from build123d import *

# Parameters (mm, degrees)
REVOLUTION_ANGLE = 180


with BuildPart() as part:
    # Sketch → Revolution (revolve)
    with BuildSketch(Plane.XY):
        Polygon((26.5, 9.5), (26.5, 17.46), (19.5, 17.46), (19.5, 18.46), (19, 18.46), (19, 28), (16.5, 28), (16.5, 9), (-19.5, 9), (-19.5, 34), (-22, 34), (-22, 26), (-40, 26), (-40, 9.5), (-50, 9.5), (-50, 2.5), (50, 2.5), (50, 9.5), align=None)
    revolve(axis=Axis((0, 0, 0), (1, 0, 0)), revolution_arc=REVOLUTION_ANGLE)


solid = part.part
For this review, take the finished solid that the model builds, in its own axes (mm). A direction names the side the tool comes from. Coordinates: 2 decimals unless noted, no trailing zeros. Order: outer loops, then holes, each group sorted by start corner. A loop starts at its lowest first (then second) coordinate and runs counter-clockwise, first axis right, second up. Notation, with made-up numbers: (53.5, 69.25) - (106.5, 69.25) arc R35 ccw to (106.5, 107.25) - close; hole circle Ø7 at (1, 46). An arc over 180 degrees is marked (long way). Answer as CSV lines item,"result". Start each with the question number.
1) Insertion check: P1, Ø3, axis at x = -14, y = -0.5, coming from the -Z side; P2, Ø6, axis at x = 26.5, z = 18.5, coming from the +Y side; P3, Ø10, axis at y = -16.5, z = 21, coming from the +X side. Each pin has a flat end and moves straight along its axis. Give the tip position at first contact, or say it passes through.
2) Machinability: for faces 1 (the cylindrical face through (-2, 0, 9)), 2 (the cylindrical face through (19.246, 0.406, 18.456)), 3 (the flat face through (-12, -8, 0)), 4 (the cylindrical face through (-31.126, 0.572, 25.994)), 5 (the flat face through (-50, 0, 5)), which of the approach directions +Z, -Z, +X, -X, +Y, -Y give a long, thin tool a straight path to every point of the face, cutting with its end or side? Answer none if there is none.
3) Add section C-C (x = 31). State the section outline as (y, z) points, then the cut area to 3 significant figures.
4) Add section A-A (z = 14). State the section outline as (x, y) points.
5) Add section B-B (y = 0). State the section outline as (x, z) points.
6) To check wall thickness, follow line 1 along X through (y, z) = (9, 17); line 2 along X through (y, z) = (15, 9.5); line 3 along X through (y, z) = (14, 25.5). State the ranges of each line that lie inside material, in increasing order. Write a range as [from, to].
7) Draft analysis for pull direction X (two halves, no side actions). For faces 6 (the flat face through (-19.5, 0, 17)), 7 (the flat face through (19.5, -2.6, 17.5)), 8 (the flat face through (-22, 2, 27)), state which applies: +X half, -X half, draft (parallel to the pull), parting line (faces both ways), or undercut.
Result:
1,P1,"z = 1.5"
1,P2,"y = 8.04"
1,P3,"x = 19"
2,face 1,"+Z"
2,face 2,"+Z, +X"
2,face 3,"-Z, +X, -X, +Y, -Y"
2,face 4,"+Z, -X"
2,face 5,"+Z, -Z, -X, +Y, -Y"
3,outline,"(-9.5, 0) - (-2.5, 0) arc R2.5 cw to (2.5, 0) - (9.5, 0) arc R9.5 ccw to start"
3,area,"132 mm^2"
4,outline,"(-40, -21.91) - (-22, -21.91) - (-22, -30.98) - (-19.5, -30.98) - (-19.5, 30.98) - (-22, 30.98) - (-22, 21.91) - (-40, 21.91) - close; (16.5, -24.25) - (19, -24.25) - (19, -12.03) - (19.5, -12.03) - (19.5, -10.43) - (26.5, -10.43) - (26.5, 10.43) - (19.5, 10.43) - (19.5, 12.03) - (19, 12.03) - (19, 24.25) - (16.5, 24.25) - close"
5,outline,"(-50, 2.5) - (50, 2.5) - (50, 9.5) - (26.5, 9.5) - (26.5, 17.46) - (19.5, 17.46) - (19.5, 18.46) - (19, 18.46) - (19, 28) - (16.5, 28) - (16.5, 9) - (-19.5, 9) - (-19.5, 34) - (-22, 34) - (-22, 26) - (-40, 26) - (-40, 9.5) - (-50, 9.5) - close"
6,line 1,"[-40, -19.5], [16.5, 19]"
6,line 2,"[-40, -19.5], [16.5, 19.5]"
6,line 3,"[-22, -19.5]"
7,face 6,"undercut"
7,face 7,"+X half"
7,face 8,"-X half"
